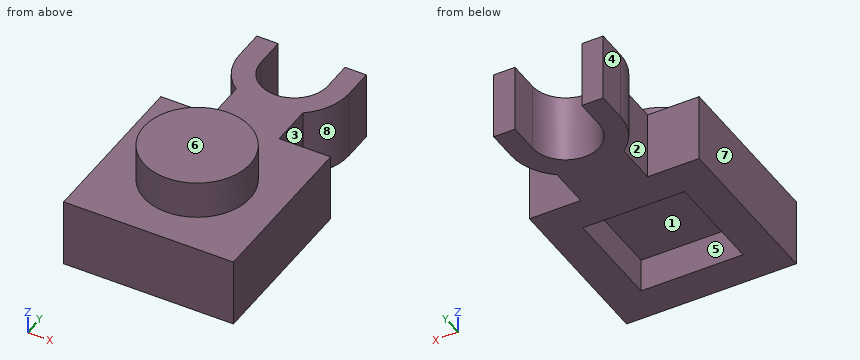
from build123d import *

# Parameters (mm, degrees)
F1_DEPTH = 3.175
F3_DEPTH = 1.7526
F4_W     = 4.7244
F4_H     = 4.7244
F5_DEPTH = 1.5748


with BuildPart() as f1:
    # F0 (on Top) → F1 (new body)
    with BuildSketch(Plane.XY):
        with BuildLine():
            Line((0, 7.874), (0, 0))
            Line((0, 0), (7.874, 0))
            Line((7.874, 0), (7.874, 7.874))
            Line((7.874, 7.874), (5.4864, 7.874))
            Line((5.4864, 7.874), (5.4864, 9.7983))
            ThreePointArc((5.4864, 9.7983), (6.215934, 10.689366), (6.477, 11.811))
            Line((6.477, 11.811), (6.477, 13.208))
            Line((6.477, 13.208), (5.4864, 13.208))
            Line((5.4864, 13.208), (5.4864, 11.811))
            ThreePointArc((5.4864, 11.811), (3.937, 10.2616), (2.3876, 11.811))
            Line((2.3876, 11.811), (2.3876, 13.208))
            Line((2.3876, 13.208), (1.397, 13.208))
            Line((1.397, 13.208), (1.397, 11.811))
            ThreePointArc((1.397, 11.811), (1.658066, 10.689366), (2.3876, 9.7983))
            Line((2.3876, 9.7983), (2.3876, 7.874))
            Line((2.3876, 7.874), (0, 7.874))
        make_face()
    extrude(amount=F1_DEPTH)

    # F2 (on face) → F3 (join)
    with BuildSketch(Plane.XY.offset(3.175)):
        with BuildLine():
            ThreePointArc((6.4008, 3.937), (3.937, 6.4008), (1.4732, 3.937))
            Line((1.4732, 3.937), (6.4008, 3.937))
        make_face()
        with BuildLine():
            Line((6.4008, 3.937), (1.4732, 3.937))
            ThreePointArc((1.4732, 3.937), (3.937, 1.4732), (6.4008, 3.937))
        make_face()
    extrude(amount=F3_DEPTH)

    # F4 (on face) → F5 (cut)
    with BuildSketch(Plane(origin=(0, 0, 0), x_dir=(1, 0, 0), z_dir=(0, 0, -1))):
        with Locations((3.937, -3.937)):
            Rectangle(F4_W, F4_H)
    extrude(amount=-F5_DEPTH, mode=Mode.SUBTRACT)


solid = f1.part
Verification items for the finished model (mm, model axes). Face numbers are marked on the shaded views. A direction names the side the tool comes from. Round coordinates to 2 decimals unless told otherwise and drop trailing zeros. Loops run counter-clockwise (first coordinate to the right, second up) from the corner with the lowest first, then second, coordinate; pieces in that order, holes last. Notation, with made-up numbers: (32, 25.25) - (77, 25.25) arc R20 cw to (77, 44.25) - close; hole circle Ø3 at (71, 30). An arc over 180 degrees is marked (long way). Use a Markdown table: item, result. Add a question column.
1. Section check C-C, the plane x = 6. Record the boundary of the cut face in (y, z) (3 decimals), plus the area to 3 significant figures.
2. Thickness scan on probe 1 along X at (y, z) = (6, 0.5); probe 2 along X at (y, z) = (12.25, 2); probe 3 along Y at (x, z) = (6, 0.85). Record the ranges inside material, lowest first. Write a range as [from, to].
3. Gauge pin test, flat ends, axial feed: pin 1 (1.1 mm diameter, centred on y = 13, z = 1, fed in from +X); pin 2 (2 mm diameter, centred on y = 9, z = 2, fed in from +X); pin 3 (1 mm diameter, centred on y = 3.5, z = 4, fed in from +X). Record the tip position at first contact, or that the pin passes through.
4. Section check A-A, the plane y = 11.5. Record the boundary of the cut face in (x, z) (3 decimals).
5. Section check D-D, the plane z = 2.65. Record the boundary of the cut face in (x, y), plus the area to 3 significant figures.
6. Section check B-B, the plane z = 0.85. Record the boundary of the cut face in (x, y), plus the area to 3 significant figures.
7. Release check for a two-part mould opening along X. For the marked faces 5, 6, 7 and 8 record: released by +X, released by -X, zero draft, split by the parting line, or undercut.
8. Access from +Z, -Z, +X, -X, +Y, -Y to the whole of each face (thin tool, end or side, straight path). Record for the marked faces 1, 2, 3 and 4.
Checks:
| question | item | result |
|---|---|---|
| 1 | outline | (0, 0) - (1.575, 0) - (1.575, 1.575) - (6.299, 1.575) - (6.299, 0) - (7.874, 0) - (7.874, 3.175) - (5.284, 3.175) - (5.284, 4.928) - (2.59, 4.928) - (2.59, 3.175) - (0, 3.175) - close; (10.329, 0) - (13.208, 0) - (13.208, 3.175) - (10.329, 3.175) - close |
| 1 | area | 31.4 mm^2 |
| 2 | probe 1 | x = [0, 1.57], [6.3, 7.87] |
| 2 | probe 2 | x = [1.4, 2.39], [5.49, 6.48] |
| 2 | probe 3 | y = [0, 1.57], [6.3, 7.87], [10.33, 13.21] |
| 3 | pin 1 | stops at x = 6.48 |
| 3 | pin 2 | stops at x = 5.72 |
| 3 | pin 3 | stops at x = 6.4 |
| 4 | outline | (1.416, 0) - (2.419, 0) - (2.419, 3.175) - (1.416, 3.175) - close; (5.455, 0) - (6.458, 0) - (6.458, 3.175) - (5.455, 3.175) - close |
| 5 | outline | (0, 0) - (7.87, 0) - (7.87, 7.87) - (5.49, 7.87) - (5.49, 9.8) arc R2.54 ccw to (6.48, 11.81) - (6.48, 13.21) - (5.49, 13.21) - (5.49, 11.81) arc R1.55 cw to (2.39, 11.81) - (2.39, 13.21) - (1.4, 13.21) - (1.4, 11.81) arc R2.54 ccw to (2.39, 9.8) - (2.39, 7.87) - (0, 7.87) - close |
| 5 | area | 76.0 mm^2 |
| 6 | outline | (0, 0) - (7.87, 0) - (7.87, 7.87) - (5.49, 7.87) - (5.49, 9.8) arc R2.54 ccw to (6.48, 11.81) - (6.48, 13.21) - (5.49, 13.21) - (5.49, 11.81) arc R1.55 cw to (2.39, 11.81) - (2.39, 13.21) - (1.4, 13.21) - (1.4, 11.81) arc R2.54 ccw to (2.39, 9.8) - (2.39, 7.87) - (0, 7.87) - close; hole (1.57, 1.57) - (6.3, 1.57) - (6.3, 6.3) - (1.57, 6.3) - close |
| 6 | area | 53.7 mm^2 |
| 7 | face 5 | undercut |
| 7 | face 6 | zero draft |
| 7 | face 7 | released by -X |
| 7 | face 8 | released by +X |
| 8 | face 1 | -Z |
| 8 | face 2 | +Z, -Z, -X |
| 8 | face 3 | +Z, -Z, +X |
| 8 | face 4 | +Z, -Z, -X, +Y |
